Read the model definition and answer for the solid it produces. Units are mm, in the model's axes. Face numbers are marked on the shaded views. A direction names the side the tool comes from. Coordinates: 2 decimals unless noted, no trailing zeros. Write each loop counter-clockwise with the first axis right and the second up, starting at its lowest first coordinate (ties: lowest second). Pieces come first, ordered by that corner, then holes.
(1) The part is cut by section C-C, the plane x = 7.5. Determine the outline of the cut face in (y, z).
(2) The part is cut by section A-A, the plane z = 2.25. Determine the outline of the cut face in (x, y) (3 decimals).
(3) Straight lines are drawn through the part: line 1 along X through (y, z) = (4.5, 0.3); line 2 along Y through (x, z) = (-15, 2.8); line 3 along Y through (x, z) = (12, 2.45). For each, find the intervals that lie inside material, in ascending order.
(4) The part is cut by section B-B, the plane y = 3. Determine the outline of the cut face in (x, z).
(5) Which of the six approach directions +Z, -Z, +X, -X, +Y, -Y give full straight-line access (tool end or side, diameter ignored) to the marked faces 1, 2, 3 and 4?
(6) Given pin 1 (1.6 mm diameter, centred on x = 9.5, z = 2.5, fed in from -Y); pin 2 (2.5 mm diameter, centred on y = 3, z = 3, fed in from -X), each flat-ended and moving along its own axis, determine where each tip first touches the part or whether it passes through.
```python
from build123d import *

# Parameters (mm, degrees)
BOSS_EXTRUDE1_DEPTH = 5.35


with BuildPart() as part:
    # Model → Boss-Extrude1 (new body)
    with BuildSketch(Plane.XY):
        with BuildLine():
            ThreePointArc((-13, 25.35), (0.467134815, 13.067225088), (16.98, 5.35))
            Line((16.98, 5.35), (6, 5.35))
            Line((6, 5.35), (6, 0))
            Line((6, 0), (-6, 0))
            Line((-6, 0), (-6, 5.35))
            Line((-6, 5.35), (-18.35, 5.35))
            Line((-18.35, 5.35), (-18.35, 18.85))
            Line((-18.35, 18.85), (-13, 18.85))
            Line((-13, 18.85), (-13, 25.35))
        make_face()
    extrude(amount=BOSS_EXTRUDE1_DEPTH)


solid = part.part
```
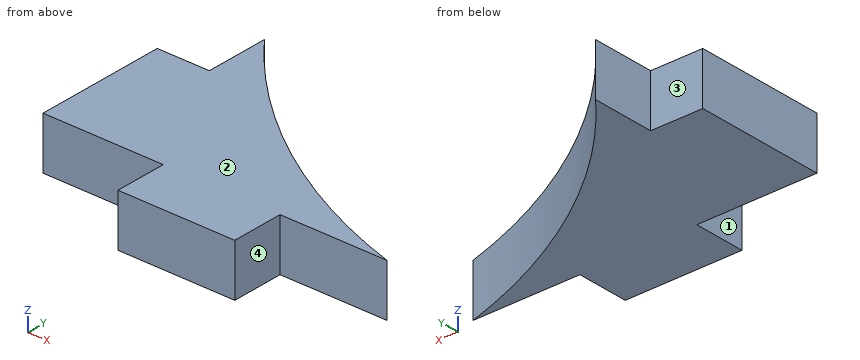
Computed:
1. outline: (5.35, 0) - (9.03, 0) - (9.03, 5.35) - (5.35, 5.35) - close
2. outline: (-18.35, 5.35) - (-6, 5.35) - (-6, 0) - (6, 0) - (6, 5.35) - (16.98, 5.35) arc R60.535 cw to (-13, 25.35) - (-13, 18.85) - (-18.35, 18.85) - close
3. line 1: x = -6 to 6
3. line 2: y = 5.35 to 18.85
3. line 3: y = 5.35 to 7.05
4. outline: (-6, 0) - (6, 0) - (6, 5.35) - (-6, 5.35) - close
5. face 1: +Z, -Z, -X, -Y
5. face 2: +Z, +X, -X, +Y, -Y
5. face 3: +Z, -Z, -X, +Y
5. face 4: +Z, -Z, +X, -Y
6. pin 1: stops at y = 5.35
6. pin 2: stops at x = -6
